Source: CAD feature listing. Evaluate the final solid. Frame: model axes, mm. Face numbers are marked on the shaded views. A direction names the side the tool comes from. Give positions to 0.01 mm unless a question says otherwise; leave off trailing zeros. Order: outer loops, then holes, each group sorted by start corner. A loop starts at its lowest first (then second) coordinate and runs counter-clockwise, first axis right, second up. Notation, with made-up numbers: M -10.5,62 L 39.5,62 A15 ccw 39.5,81 Z; hole C 68,26 d1. An arc over 180 degrees is marked long. Answer in a Markdown table with one row per item. Add a question column.
(1) Mould query, pull axis X, two halves, no side actions, for the marked faces 3, 4, 5 and 6. Classes: pulls with the +X half, pulls with the -X half, needs draft (parallel to the pull), parting line crosses it, or undercut.
(2) Section query B-B, the plane x = -14. Return loops of the section in (y, z), plus the area to 3 significant figures.
(3) Section query A-A, the plane y = 0. Return loops of the section in (x, z), plus the area to 3 significant figures.
(4) Material intervals for line 1 along Y through (x, z) = (0, 5.5); line 2 along Y through (x, z) = (4, 6.75); line 3 along X through (y, z) = (15, 3), sorted ascending.
(5) Section query C-C, the plane y = -34. Return loops of the section in (x, z), plus the area to 3 significant figures.
(6) Section query D-D, the plane x = 1.5. Return loops of the section in (y, z), plus the area to 3 significant figures.
(7) Pin query (flat end, axial travel): P1, Ø13, axis at x = 0, y = 0, coming from the -Z side; P2, Ø3, axis at x = 24.5, z = 4, coming from the -Y side; P3, Ø1, axis at x = 24.5, z = 5.5, coming from the +Y side; P4, Ø1, axis at y = -27, z = 3.5, coming from the +X side. Return the tip coordinate at first contact, or that it passes through.
(8) Set-up query: the marked faces 1 and 2. Return all of +Z, -Z, +X, -X, +Y, -Y with unobstructed straight access to the full face (end or side cutting, diameter ignored); none if empty.
from build123d import *

# Parameters (mm, degrees)
F0_R     = 11
F1_DEPTH = 7
F2_D     = 22


with BuildPart() as f1:
    # F0 (on Top) → F1 (new body)
    with BuildSketch(Plane.XY):
        with BuildLine():
            Line((16.352598, -29.827668), (5.998279, -11.893462))
            Line((5.998279, -11.893462), (4.426611, -12.544469))
            Line((4.426611, -12.544469), (13.431306, -28.141059))
            ThreePointArc((13.431306, -28.141059), (13.431306, -34.491059), (7.932045, -37.666059))
            Line((7.932045, -37.666059), (-8.176027, -37.666059))
            ThreePointArc((-8.176027, -37.666059), (-13.675289, -34.491059), (-13.675289, -28.141059))
            Line((-13.675289, -28.141059), (-4.623506, -12.462912))
            Line((-4.623506, -12.462912), (-6.195175, -11.811905))
            Line((-6.195175, -11.811905), (-16.59658, -29.827668))
            ThreePointArc((-16.59658, -29.827668), (-16.59658, -36.177668), (-11.097319, -39.352668))
            Line((-11.097319, -39.352668), (10.853336, -39.352668))
            ThreePointArc((10.853336, -39.352668), (16.352598, -36.177668), (16.352598, -29.827668))
        make_face()
        with BuildLine():
            Line((30.836118, 16.474589), (12.047307, 5.626864))
            Line((12.047307, 5.626864), (12.698314, 4.055195))
            Line((12.698314, 4.055195), (14.378031, 0))
            Line((14.378031, 0), (12.698314, -4.055195))
            Line((12.698314, -4.055195), (12.047307, -5.626864))
            Line((12.047307, -5.626864), (30.836118, -16.474589))
            ThreePointArc((30.836118, -16.474589), (37.186118, -16.474589), (40.361118, -10.975328))
            Line((40.361118, -10.975328), (40.361118, 10.975328))
            ThreePointArc((40.361118, 10.975328), (37.186118, 16.474589), (30.836118, 16.474589))
        make_face()
        with BuildLine():
            Line((-12.698314, 4.055195), (-12.047307, 5.626864))
            Line((-12.047307, 5.626864), (-30.836118, 16.474589))
            ThreePointArc((-30.836118, 16.474589), (-37.186118, 16.474589), (-40.361118, 10.975328))
            Line((-40.361118, 10.975328), (-40.361118, -10.975328))
            ThreePointArc((-40.361118, -10.975328), (-37.186118, -16.474589), (-30.836118, -16.474589))
            Line((-30.836118, -16.474589), (-12.047307, -5.626864))
            Line((-12.047307, -5.626864), (-12.698314, -4.055195))
            Line((-12.698314, -4.055195), (-29.149509, -13.553298))
            ThreePointArc((-29.149509, -13.553298), (-35.499509, -13.553298), (-38.674509, -8.054036))
            Line((-38.674509, -8.054036), (-38.674509, 8.054036))
            ThreePointArc((-38.674509, 8.054036), (-35.499509, 13.553298), (-29.149509, 13.553298))
            Line((-29.149509, 13.553298), (-12.698314, 4.055195))
        make_face()
        with BuildLine():
            Line((13.431306, -28.141059), (4.426611, -12.544469))
            Line((4.426611, -12.544469), (0, -14.378031))
            Line((0, -14.378031), (-4.623506, -12.462912))
            Line((-4.623506, -12.462912), (-13.675289, -28.141059))
            ThreePointArc((-13.675289, -28.141059), (-13.675289, -34.491059), (-8.176027, -37.666059))
            Line((-8.176027, -37.666059), (7.932045, -37.666059))
            ThreePointArc((7.932045, -37.666059), (13.431306, -34.491059), (13.431306, -28.141059))
        make_face()
        Polygon((5.998279, 11.893462), (0, 14.378031), (-6.195175, 11.811905), (-10.166803, 10.166803), (-12.047307, 5.626864), (-12.698314, 4.055195), (-14.378031, 0), (-12.698314, -4.055195), (-12.047307, -5.626864), (-10.166803, -10.166803), (-6.195175, -11.811905), (-4.623506, -12.462912), (0, -14.378031), (4.426611, -12.544469), (5.998279, -11.893462), (10.166803, -10.166803), (12.047307, -5.626864), (12.698314, -4.055195), (14.378031, 0), (12.698314, 4.055195), (12.047307, 5.626864), (10.166803, 10.166803), align=None)
        Circle(F0_R, mode=Mode.SUBTRACT)
        with BuildLine():
            Line((-6.195175, 11.811905), (0, 14.378031))
            Line((0, 14.378031), (5.998279, 11.893462))
            Line((5.998279, 11.893462), (16.352598, 29.827668))
            ThreePointArc((16.352598, 29.827668), (16.352598, 36.177668), (10.853336, 39.352668))
            Line((10.853336, 39.352668), (-11.097319, 39.352668))
            ThreePointArc((-11.097319, 39.352668), (-16.59658, 36.177668), (-16.59658, 29.827668))
            Line((-16.59658, 29.827668), (-6.195175, 11.811905))
        make_face()
        with BuildLine():
            Line((-14.378031, 0), (-12.698314, 4.055195))
            Line((-12.698314, 4.055195), (-29.149509, 13.553298))
            ThreePointArc((-29.149509, 13.553298), (-35.499509, 13.553298), (-38.674509, 8.054036))
            Line((-38.674509, 8.054036), (-38.674509, -8.054036))
            ThreePointArc((-38.674509, -8.054036), (-35.499509, -13.553298), (-29.149509, -13.553298))
            Line((-29.149509, -13.553298), (-12.698314, -4.055195))
            Line((-12.698314, -4.055195), (-14.378031, 0))
        make_face()
        Circle(F0_R)
    extrude(amount=F1_DEPTH)

    # F2 (through all)
    with Locations(Plane(origin=(0, 0, 0), x_dir=(1, 0, 0), z_dir=(0, 0, -1))):
        with Locations((-27.674509, 0), (-0.121991, -26.666059), (0, 0), (27.674509, 0), (-0.121991, 26.666059)):
            Hole(F2_D / 2)


solid = f1.part
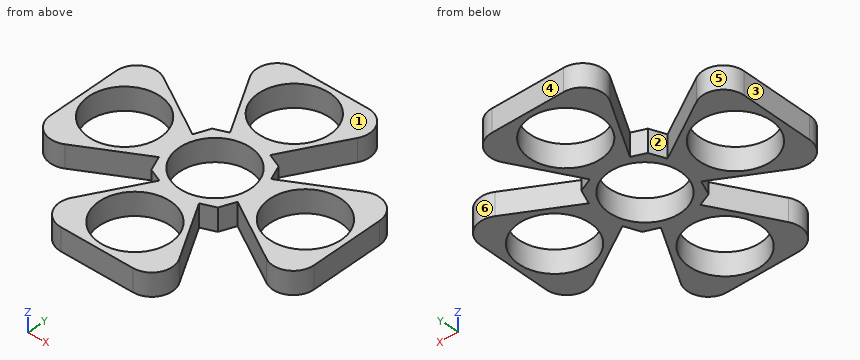
Values follow:
| question | item | result |
|---|---|---|
| 1 | face 3 | pulls with the -X half |
| 1 | face 4 | needs draft |
| 1 | face 5 | undercut |
| 1 | face 6 | undercut |
| 2 | outline | M -38.65,0 L -25.33,0 L -25.33,7 L -38.65,7 Z; M -6.75,0 L 6.75,0 L 6.75,7 L -6.75,7 Z; M 25.33,0 L 38.65,0 L 38.65,7 L 25.33,7 Z |
| 2 | area | 281 mm² |
| 3 | outline | M -40.36,0 L -38.67,0 L -38.67,7 L -40.36,7 Z; M -16.67,0 L -11,0 L -11,7 L -16.67,7 Z; M 11,0 L 16.67,0 L 16.67,7 L 11,7 Z; M 38.67,0 L 40.36,0 L 40.36,7 L 38.67,7 Z |
| 3 | area | 103 mm² |
| 4 | line 1 | y = -39.35 to -37.67, -15.67 to -11, 11 to 15.67, 37.67 to 39.35 |
| 4 | line 2 | y = -39.35 to -36.86, -16.47 to -10.25, 10.25 to 16.47, 36.86 to 39.35 |
| 4 | line 3 | x = -38.92 to -28.28, -8.04 to 7.79, 28.28 to 38.92 |
| 5 | outline | M -17.37,0 L -8.32,0 L -8.32,7 L -17.37,7 Z; M 8.08,0 L 17.12,0 L 17.12,7 L 8.08,7 Z |
| 5 | area | 127 mm² |
| 6 | outline | M -39.35,0 L -37.55,0 L -37.55,7 L -39.35,7 Z; M -15.79,0 L -10.9,0 L -10.9,7 L -15.79,7 Z; M 10.9,0 L 15.79,0 L 15.79,7 L 10.9,7 Z; M 37.55,0 L 39.35,0 L 39.35,7 L 37.55,7 Z |
| 6 | area | 93.7 mm² |
| 7 | P1 | passes through |
| 7 | P2 | stops at y = -13.68 |
| 7 | P3 | stops at y = 13.11 |
| 7 | P4 | stops at x = 15.01 |
| 8 | face 1 | +Z, +X, -X, +Y, -Y |
| 8 | face 2 | +Z, -Z |
